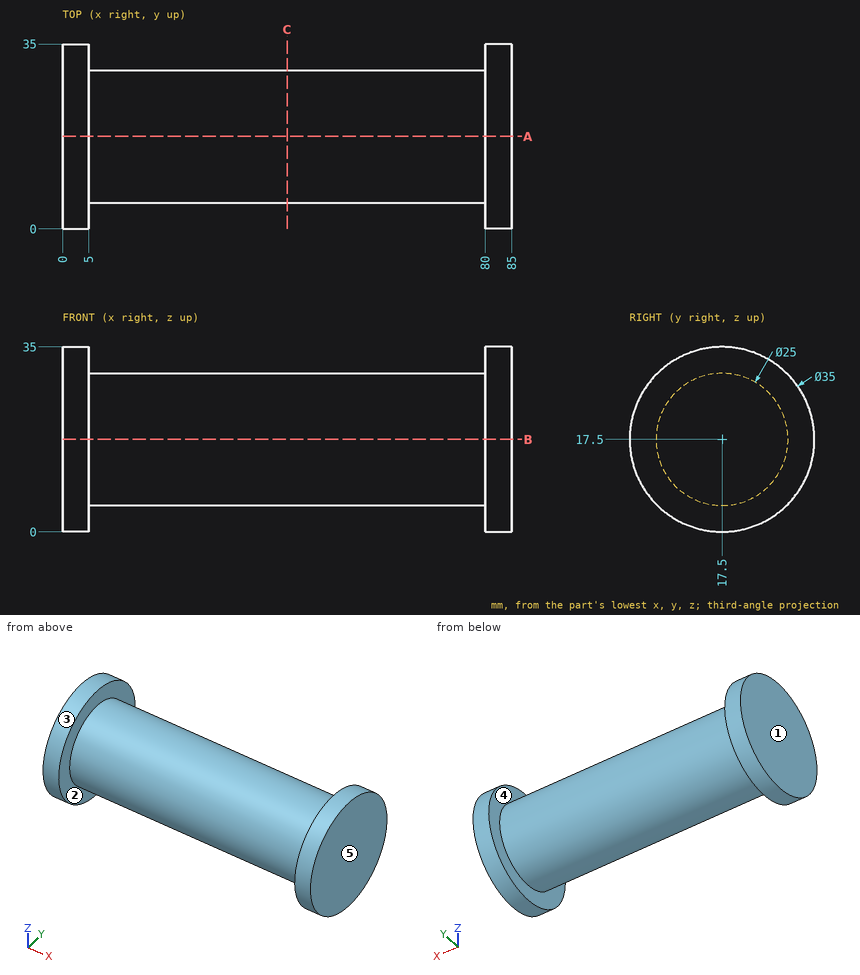
Study the drawing (mm; zero at the part's minimum x, y, z) and answer. A direction names the side the tool comes from. Give positions to 0.01 mm unless a question says otherwise; leave off trailing zeros. Write each loop counter-clockwise with the first axis right and the second up, starting at its lowest first coordinate (ties: lowest second). Pieces come first, ordered by that corner, then holes.
Item 1: Which of the six approach directions +Z, -Z, +X, -X, +Y, -Y give full straight-line access (tool end or side, diameter ignored) to the marked faces 1 and 2?
Item 2: Section A-A, the plane y = 17.5 is taken. Write down the section's boundary in (x, z).
Item 3: Section C-C, the plane x = 42.5 is taken. Write down the section's boundary in (y, z), plus the area to 3 significant figures.
Item 4: Determine the mould class of the marked faces 3, 4 and 5 for opening direction X: released by +X, released by -X, zero draft, split by the parting line, or undercut.
Item 5: Find the intervals of material crossed by line 1 along X through (y, z) = (20, 32); line 2 along Y through (x, z) = (56.5, 17.5); line 3 along Y through (x, z) = (74, 7.5), in increasing order.
Item 6: Flat-ended cylindrical pins translate along their axes: P1, Ø12, axis at x = 61, y = 26, coming from the +Z side; P2, Ø5, axis at x = 18, z = 7.5, coming from the +Y side; P3, Ø1, axis at x = 18, z = 12.5, coming from the -Y side. Find the tip coordinate at first contact, or state that the pin passes through.
Completed:
1. face 1: +Z, -Z, -X, +Y, -Y
1. face 2: none
2. outline: (0, 0) - (5, 0) - (5, 5) - (80, 5) - (80, 0) - (85, 0) - (85, 35) - (80, 35) - (80, 30) - (5, 30) - (5, 35) - (0, 35) - close
3. outline: circle Ø25 at (17.5, 17.5)
3. area: 491 mm2
4. face 3: zero draft
4. face 4: undercut
4. face 5: released by +X
5. line 1: x = 0 to 5, 80 to 85
5. line 2: y = 5 to 30
5. line 3: y = 10 to 25
6. P1: stops at z = 29.75
6. P2: stops at y = 27.5
6. P3: stops at y = 5.84
